For this review, take the finished solid that the model builds, in its own axes (mm). A direction names the side the tool comes from. Round coordinates to 2 decimals unless told otherwise and drop trailing zeros. Order: outer loops, then holes, each group sorted by start corner. A loop starts at its lowest first (then second) coordinate and runs counter-clockwise, first axis right, second up. Notation, with made-up numbers: M 28,51.25 L 56,51.25 A24 ccw 56,66.25 Z; hole C -13.5,42.25 d6. An arc over 180 degrees is marked long. Put each result on its own line as item: value.
from build123d import *

# Parameters (mm, degrees)
ESBO_O1_R                = 1.25
RESSALTO_EXTRUS_O1_DEPTH = 2
ESBO_O2_R                = 0.75
RESSALTO_EXTRUS_O2_DEPTH = 5
ESBO_O3_R                = 1.75
RESSALTO_EXTRUS_O3_DEPTH = 4


with BuildPart() as part:
    # Esboço1 → Ressalto-extrusão1 (new body)
    with BuildSketch(Plane.XY):
        with BuildLine():
            Line((-27, 4), (27, 4))
            ThreePointArc((27, 4), (31, 0), (27, -4))
            Line((27, -4), (-27, -4))
            ThreePointArc((-27, -4), (-31, 0), (-27, 4))
        make_face()
        with Locations((23, -2.5)):
            Circle(ESBO_O1_R, mode=Mode.SUBTRACT)
        with BuildLine():
            Line((-27, 1.4), (-7, 1.4))
            ThreePointArc((-7, 1.4), (-5.6, 0), (-7, -1.4))
            Line((-7, -1.4), (-27, -1.4))
            ThreePointArc((-27, -1.4), (-28.4, 0), (-27, 1.4))
        make_face(mode=Mode.SUBTRACT)
    extrude(amount=RESSALTO_EXTRUS_O1_DEPTH)

    # Esboço2 → Ressalto-extrusão2 (add)
    with BuildSketch(Plane.XY.offset(2)):
        with Locations((27, -2.4)):
            Circle(ESBO_O2_R)
    extrude(amount=-RESSALTO_EXTRUS_O2_DEPTH)

    # Esboço3 → Ressalto-extrusão3 (add)
    with BuildSketch(Plane(origin=(0, 0, 0), x_dir=(0, 0, -1), z_dir=(1, 0, 0))):
        with BuildLine():
            Line((-2, 4), (-2, 11))
            ThreePointArc((-2, 11), (5.96386061, 14.497656355), (3.150989464, 6.266955795))
            Line((3.150989464, 6.266955795), (0, 6))
            Line((0, 6), (0, 4))
            Line((0, 4), (-2, 4))
        make_face()
        with Locations((2.75, 11)):
            Circle(ESBO_O3_R, mode=Mode.SUBTRACT)
    extrude(amount=RESSALTO_EXTRUS_O3_DEPTH)


solid = part.part
(1) Add section D-D on z = -6.75. Give the boundary of the cut face in (x, y).
A:
outline: M 0,8.44 L 4,8.44 L 4,13.56 L 0,13.56 Z
(2) Add section C-C on z = 1.25. Give the boundary of the cut face in (x, y).
A:
outline: M -27,-4 L 27,-4 A4 ccw 27,4 L 4,4 L 4,13.56 L 0,13.56 L 0,4 L -27,4 A4 ccw Z; hole M -27,-1.4 L -7,-1.4 A1.4 ccw -7,1.4 L -27,1.4 A1.4 ccw Z; hole C 23,-2.5 d2.5
(3) Insertion check: pin 1 Ø2 at (x, y) = (-15, 0.5) entering from +Z; pin 2 Ø10 at (x, y) = (0, -1.5) entering from -Z; pin 3 Ø3 at (y, z) = (11, -2.75) entering from +X; pin 4 Ø2 at (x, z) = (-19.5, 1.5) entering from +Y. Each pin has a flat end and moves straight along its axis. Give the tip position at first contact, or say it passes through.
A:
pin 1: stops at z = 2
pin 2: stops at z = 0
pin 3: passes through
pin 4: stops at y = 4
(4) For faces 5 (the face through (4, 11.3, -0.7)), 6 (the face through (0, 11.3, -0.7)), 7 (the face through (1.972, 6.135, -1.598)), 8 (the face through (-17, 1.4, 1)), list the 3-axis set-ups (+Z, -Z, +X, -X, +Y, -Y) from which the entire face can be reached by the end or side of a thin tool; tool diameter is ignored.
A:
face 5: +Z, -Z, +X, +Y
face 6: +Z, -Z, -X, +Y
face 7: -Z, +X, -X, -Y
face 8: +Z, -Z
(5) To check wall thickness, follow L1, parallel to Y at x = 23, z = 1.55; L2, parallel to Y at x = -15, z = 1.75; L3, parallel to X at y = 6.75, z = -1.75. State the ranges of each line that lie inside material, in increasing order.
A:
L1: y = -4 to -3.75, -1.25 to 4
L2: y = -4 to -1.4, 1.4 to 4
L3: x = 0 to 4
(6) Draft analysis for pull direction X (two halves, no side actions). For faces 1 (the face through (-31, 0, 1)), 2 (the face through (27.715, -2.175, -1.479)), 3 (the face through (0, -4, 1)), 4 (the face through (24.155, -2.979, 0.986)), state which applies: released by +X, released by -X, zero draft, split by the parting line, or undercut.
A:
face 1: released by -X
face 2: split by the parting line
face 3: zero draft
face 4: undercut
(7) Add section B-B on y = 0.25. Give the boundary of the cut face in (x, z), then the cut area to 3 significant figures.
A:
outline: M -30.99,0 L -28.38,0 L -28.38,2 L -30.99,2 Z; M -5.62,0 L 30.99,0 L 30.99,2 L -5.62,2 Z
area: 78.5 mm2
(8) Add section A-A on x = 23. Give the boundary of the cut face in (y, z).
A:
outline: M -4,0 L -3.75,0 L -3.75,2 L -4,2 Z; M -1.25,0 L 4,0 L 4,2 L -1.25,2 Z
